Here's how the part is built. I have some questions about the finished solid (model axes, mm). A direction names the side the tool comes from. Give positions to 0.01 mm unless a question says otherwise; leave off trailing zeros. Loops run counter-clockwise (first coordinate to the right, second up) from the corner with the lowest first, then second, coordinate; pieces in that order, holes last. Notation, with made-up numbers: (44.25, 22) - (67.25, 22) arc R23 ccw to (67.25, 57) - close; hole circle Ø2 at (88, 40.25). An arc over 180 degrees is marked (long way). Use a Markdown table: item, result.
from build123d import *

# Parameters (mm, degrees)
SKETCH1_W           = 100
SKETCH1_H           = 25
BOSS_EXTRUDE1_DEPTH = 15
SKETCH2_W           = 100
SKETCH2_H           = 5
SKETCH2_W_2         = 10
SKETCH2_H_2         = 2
BOSS_EXTRUDE2_DEPTH = 2


with BuildPart() as part:
    # Sketch1 → Boss-Extrude1 (new body)
    with BuildSketch(Plane.XY):
        Polygon((0, 0), (0, 33), (100, 33), (100, 0), (102, 0), (102, 62), (-2, 62), (-2, 0), align=None)
        with Locations((50, 47.5)):
            Rectangle(SKETCH1_W, SKETCH1_H, mode=Mode.SUBTRACT)
    extrude(amount=BOSS_EXTRUDE1_DEPTH)

    # Sketch2 → Boss-Extrude2 (add)
    # profile 1 of 2: a face of its own
    with BuildSketch(Plane(origin=(0, 0, 15), x_dir=(-1, 0, 0), z_dir=(0, 0, -1))):
        with Locations((-50, 57.5)):
            Rectangle(SKETCH2_W, SKETCH2_H)
        with Locations((-74, 57.5)):
            Rectangle(SKETCH2_W_2, SKETCH2_H_2, mode=Mode.SUBTRACT)
        with Locations((-90, 57.5)):
            Rectangle(SKETCH2_W_2, SKETCH2_H_2, mode=Mode.SUBTRACT)
        with Locations((-58, 57.5)):
            Rectangle(SKETCH2_W_2, SKETCH2_H_2, mode=Mode.SUBTRACT)
        with Locations((-42, 57.5)):
            Rectangle(SKETCH2_W_2, SKETCH2_H_2, mode=Mode.SUBTRACT)
        with Locations((-26, 57.5)):
            Rectangle(SKETCH2_W_2, SKETCH2_H_2, mode=Mode.SUBTRACT)
        with Locations((-10, 57.5)):
            Rectangle(SKETCH2_W_2, SKETCH2_H_2, mode=Mode.SUBTRACT)
    # profile 2 of 2: a face of its own
    with BuildSketch(Plane(origin=(0, 0, 15), x_dir=(-1, 0, 0), z_dir=(0, 0, -1))):
        with Locations((-50, 30.5)):
            Rectangle(SKETCH2_W, SKETCH2_H)
        with Locations((-74, 30.5)):
            Rectangle(SKETCH2_W_2, SKETCH2_H_2, mode=Mode.SUBTRACT)
        with Locations((-90, 30.5)):
            Rectangle(SKETCH2_W_2, SKETCH2_H_2, mode=Mode.SUBTRACT)
        with Locations((-58, 30.5)):
            Rectangle(SKETCH2_W_2, SKETCH2_H_2, mode=Mode.SUBTRACT)
        with Locations((-42, 30.5)):
            Rectangle(SKETCH2_W_2, SKETCH2_H_2, mode=Mode.SUBTRACT)
        with Locations((-26, 30.5)):
            Rectangle(SKETCH2_W_2, SKETCH2_H_2, mode=Mode.SUBTRACT)
        with Locations((-10, 30.5)):
            Rectangle(SKETCH2_W_2, SKETCH2_H_2, mode=Mode.SUBTRACT)
    extrude(amount=BOSS_EXTRUDE2_DEPTH)


solid = part.part
(1) Will these pins go through, and if not, where does the flat tip stop? pin 1 (0.6 mm diameter, centred on x = 44.5, z = 14, fed in from -Y); pin 2 (1.5 mm diameter, centred on x = 57.5, y = 56.5, fed in from -Z); pin 3 (10 mm diameter, centred on x = 23, y = 49, fed in from +Z).
A:
| item | result |
|---|---|
| pin 1 | y = 28 |
| pin 2 | z = 13 |
| pin 3 | through |
(2) On a 3-axis mill with a long thin cutter (end or side, diameter ignored), from which of +Z, -Z, +X, -X, +Y, -Y can I reach the whole of each face in a straight line? I mean faces 4 (the face through (85, 30, 14)), 5 (the face through (34.3, 33.4, 0)), 6 (the face through (51, 31, 13)). Say none if no direction works.
A:
| item | result |
|---|---|
| face 4 | +Z, -Z |
| face 5 | -Z, +X, -X, +Y, -Y |
| face 6 | -Z, -Y |
(3) If I drill on line 1 (Y direction, x = 77, z = 13.5); line 2 (Y direction, x = 60, z = 9.5); line 3 (X direction, y = 3.5, z = 12), over which ranges is the centre line in solid material (lowest first)?
A:
| item | result |
|---|---|
| line 1 | 28 to 29.5, 31.5 to 35, 55 to 56.5, 58.5 to 62 |
| line 2 | 33 to 35, 60 to 62 |
| line 3 | -2 to 0, 100 to 102 |
(4) Suppose I cut it at A-A on x = 59. Write out the boundary of the cut face in (y, z).
A:
| item | result |
|---|---|
| outline | (28, 13) - (29.5, 13) - (29.5, 15) - (28, 15) - close; (31.5, 13) - (33, 13) - (33, 0) - (35, 0) - (35, 15) - (31.5, 15) - close; (55, 13) - (56.5, 13) - (56.5, 15) - (55, 15) - close; (58.5, 13) - (60, 13) - (60, 0) - (62, 0) - (62, 15) - (58.5, 15) - close |
(5) Suppose I cut it at D-D on y = 21. Write out the boundary of the cut face in (x, z), plus the area to 3 significant figures.
A:
| item | result |
|---|---|
| outline | (-2, 0) - (0, 0) - (0, 15) - (-2, 15) - close; (100, 0) - (102, 0) - (102, 15) - (100, 15) - close |
| area | 60.0 mm2 |
(6) Suppose I cut it at C-C on z = 2.25. Write out the boundary of the cut face in (x, y).
A:
| item | result |
|---|---|
| outline | (-2, 0) - (0, 0) - (0, 33) - (100, 33) - (100, 0) - (102, 0) - (102, 62) - (-2, 62) - close; hole (0, 35) - (100, 35) - (100, 60) - (0, 60) - close |
(7) We'd pull the mould along Y, two halves only. Please class faces 1 (the face through (51, 62, 7)), 2 (the face through (101, 0, 7)), 3 (the face through (58, 29.5, 14)): pulls with the +Y half, pulls with the -Y half, needs draft (parallel to the pull), parting line crosses it, or undercut.
A:
| item | result |
|---|---|
| face 1 | pulls with the +Y half |
| face 2 | pulls with the -Y half |
| face 3 | undercut |
(8) Suppose I cut it at B-B on y = 30.5. Count the separate pieces of the cut face and the enclosed holes in it, plus the area to 3 significant figures.
A:
| item | result |
|---|---|
| separate pieces | 7 |
| enclosed holes | 0 |
| area | 140 mm2 |
